Autodesk Inventor part; units mm, degrees
ref_plane "YZ Plane" through (0, 0, 0) normal (1, 0, 0) x (0, 1, 0)
ref_plane "XZ Plane" through (0, 0, 0) normal (0, 1, 0) x (-1, 0, 0)
ref_plane "XY Plane" through (0, 0, 0) normal (0, 0, 1) x (1, 0, 0)
sketch "Sketch1" plane through (0, 0, 0) normal (0, 1, 0) x (-1, 0, 0)
  circle A0 centre (0, 0) radius 4
  dimension "d0" = 8
extrude "Extrusion1" add sketch "Sketch1" along normal blind 3
sketch "Sketch2" plane through (0, 3, 0) normal (0, 1, 0) x (1, 0, 0)
  circle A0 centre (0, 0) radius 2
  dimension "d3" = 4
extrude "Extrusion2" add sketch "Sketch2" along normal blind 8.5
sketch "Sketch3" plane through (0, 11.5, 0) normal (0, 1, 0) x (1, 0, 0)
  point P0 (0, 0)
hole "Hole1" at (0, 11.5, 0) direction (0, -1, 0) diameter 3.1 end through all
properties part number "Tensioner"
The listing builds one solid part. Answer for the finished solid, in the listing's coordinates (mm). Coordinates: 2 decimals unless noted, no trailing zeros. Order: outer loops, then holes, each group sorted by start corner. A loop starts at its lowest first (then second) coordinate and runs counter-clockwise, first axis right, second up.
Q1. Consider line 1 (X direction, y = 4.75, z = 0); line 2 (Y direction, x = 1.5, z = -3). Determine where each line is inside the solid, lowest interval first.
Q2. A cutting plane is placed at C-C, the plane y = 10.5. Write down the section's boundary in (x, z).
Q3. Given P1, Ø4, axis at x = 1.5, z = -2, coming from the +Y side; P2, Ø3, axis at x = -0.5, y = 9.5, coming from the +Z side; P3, Ø1, axis at y = 7.5, z = 0, coming from the -X side; P4, Ø2, axis at x = 2, y = 7, coming from the -Z side, each flat-ended and moving along its own axis, determine where each tip first touches the part or whether it passes through.
Q4. A cutting plane is placed at B-B, the plane z = 0. Write down the section's boundary in (x, y), and give its area (4 significant figures).
Q5. A cutting plane is placed at D-D, the plane x = -3. Write down the section's boundary in (y, z).
Q6. A cutting plane is placed at A-A, the plane x = 0. Write down the section's boundary in (y, z).
Q7. For a pull along Z with two mould halves and no side action, classify faces 1 (the face through (-2, 0, 0)), 2 (the face through (0.867, 1.479, 3.905)), 3 (the face through (1.375, 5.67, 0.715)) as pulls with the +Z half, pulls with the -Z half, needs draft (parallel to the pull), parting line crosses it, or undercut.
Answers follow:
1. line 1: x = -2 to -1.55, 1.55 to 2
1. line 2: y = 0 to 3
2. outline: circle Ø4 at (0, 0); hole circle Ø3.1 at (0, 0)
3. P1: stops at y = 11.5
3. P2: stops at z = 2
3. P3: stops at x = -2
3. P4: stops at z = -1.73
4. outline: (-4, 0) - (-1.55, 0) - (-1.55, 11.5) - (-2, 11.5) - (-2, 3) - (-4, 3) - close; (1.55, 0) - (4, 0) - (4, 3) - (2, 3) - (2, 11.5) - (1.55, 11.5) - close
4. area: 22.35 mm2
5. outline: (0, -2.65) - (3, -2.65) - (3, 2.65) - (0, 2.65) - close
6. outline: (0, -4) - (3, -4) - (3, -2) - (11.5, -2) - (11.5, -1.55) - (0, -1.55) - close; (0, 1.55) - (11.5, 1.55) - (11.5, 2) - (3, 2) - (3, 4) - (0, 4) - close
7. face 1: needs draft
7. face 2: parting line crosses it
7. face 3: undercut
